```python
from build123d import *

# Parameters (mm, degrees)
F0_W           = 90
F0_H           = 60
F1_DEPTH       = 10
F3_D           = 4.5
F3_CBORE_D     = 8
F3_CBORE_DEPTH = 4.4
F5_D           = 5
F7_D           = 3.3


with BuildPart() as f1:
    # F0 (on Top) → F1 (new body)
    with BuildSketch(Plane.XY):
        Rectangle(F0_W, F0_H)
    extrude(amount=F1_DEPTH)

    # F3 (through all)
    with Locations(Plane.XY.offset(10)):
        with Locations((-38, 12.9876444116), (-17, -13.0123555884)):
            CounterBoreHole(F3_D / 2, F3_CBORE_D / 2, F3_CBORE_DEPTH)

    # F5 (through all)
    with Locations(Plane.XY.offset(10)):
        with Locations((-38, -13), (-17, 13)):
            Hole(F5_D / 2)

    # F7 (through all)
    with Locations(Plane.XY.offset(10)):
        with Locations((37, 22.5), (37, -22.5)):
            Hole(F7_D / 2)


solid = f1.part
```
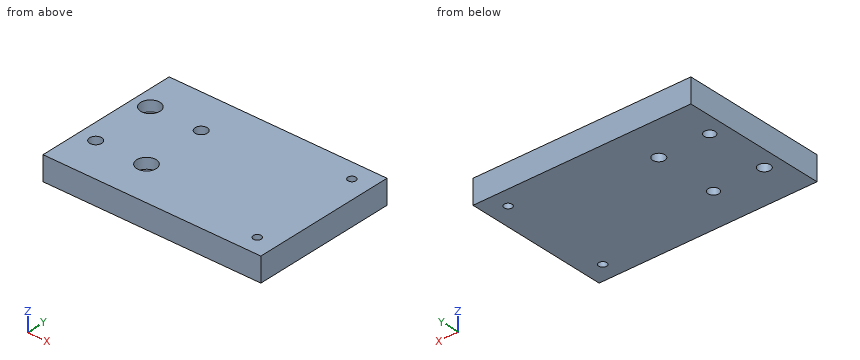
For this review, take the finished solid that the model builds, in its own axes (mm). Coordinates: 2 decimals unless noted, no trailing zeros. Order: outer loops, then holes, each group sorted by start corner. A loop starts at its lowest first (then second) coordinate and runs counter-clockwise, first axis right, second up. Notation, with made-up numbers: (39.5, 82) - (86.5, 82) arc R20 ccw to (86.5, 100) - close; hole circle Ø10 at (-11.5, 81). An arc over 180 degrees is marked (long way). Answer as a JSON object with one key per item and string values. Group by question number.
1. We need section D-D on y = 12. State the section outline as (x, z) points.
2. For probe 1 along Y at (x, z) = (-38, 2.5); probe 2 along Y at (x, z) = (-17, 5); probe 3 along X at (y, z) = (-13.5, 9.25), list the stretches that pass through material, from the lowest coordinate up.
3. We need section B-B on y = -22.5. State the section outline as (x, z) points, then the cut area to 3 significant figures.
4. We need section C-C on z = 3.25. State the section outline as (x, y) points.
5. We need section A-A on x = -17. State the section outline as (y, z) points.
6. Clearance check with flat-ended pins moving along their axes: P1, Ø6, axis at x = -38, y = 12.99, coming from the -Z side; P2, Ø2.5, axis at x = -17, y = -13.01, coming from the +Z side. State where each tip first meets the part, or that it passes through.
Final values:
{
 "1": {"outline": "(-45, 0) - (-40.02, 0) - (-40.02, 5.6) - (-41.88, 5.6) - (-41.88, 10) - (-45, 10) - close; (-35.98, 0) - (-19.29, 0) - (-19.29, 10) - (-34.12, 10) - (-34.12, 5.6) - (-35.98, 5.6) - close; (-14.71, 0) - (45, 0) - (45, 10) - (-14.71, 10) - close"},
 "2": {"probe 1": "-30 to -15.5, -10.5 to 10.74, 15.24 to 30", "probe 2": "-30 to -15.26, -10.76 to 10.5, 15.5 to 30", "probe 3": "-45 to -40.45, -35.55 to -20.97, -13.03 to 45"},
 "3": {"outline": "(-45, 0) - (35.35, 0) - (35.35, 10) - (-45, 10) - close; (38.65, 0) - (45, 0) - (45, 10) - (38.65, 10) - close", "area": "867 mm²"},
 "4": {"outline": "(-45, -30) - (45, -30) - (45, 30) - (-45, 30) - close; hole circle Ø5 at (-38, -13); hole circle Ø4.5 at (-38, 12.99); hole circle Ø5 at (-17, 13); hole circle Ø4.5 at (-17, -13.01); hole circle Ø3.3 at (37, -22.5); hole circle Ø3.3 at (37, 22.5)"},
 "5": {"outline": "(-30, 0) - (-15.26, 0) - (-15.26, 5.6) - (-17.01, 5.6) - (-17.01, 10) - (-30, 10) - close; (-10.76, 0) - (10.5, 0) - (10.5, 10) - (-9.01, 10) - (-9.01, 5.6) - (-10.76, 5.6) - close; (15.5, 0) - (30, 0) - (30, 10) - (15.5, 10) - close"},
 "6": {"P1": "z = 0", "P2": "through"}
}
